```python
from build123d import *

# Parameters (mm, degrees)
SKETCH3_W           = 170.58
SKETCH3_H           = 100
BOSS_EXTRUDE1_DEPTH = 5
SKETCH4_W           = 5
SKETCH4_H           = 100
BOSS_EXTRUDE2_DEPTH = 24.94
SKETCH6_W           = 160.58
SKETCH6_H           = 5
BOSS_EXTRUDE3_DEPTH = 24.94
BOSS_EXTRUDE4_DEPTH = 24.94
SKETCH8_R           = 1.75
CUT_EXTRUDE1_DEPTH  = 8
SKETCH9_W           = 7.75
SKETCH9_H           = 6.74
CUT_EXTRUDE2_DEPTH  = 10
CUT_EXTRUDE3_DEPTH  = 10
SKETCH11_R          = 1.75
CUT_EXTRUDE4_DEPTH  = 10
SKETCH13_W          = 40.2
SKETCH13_H          = 14.565
CUT_EXTRUDE6_DEPTH  = 200
SKETCH14_R          = 1.75
CUT_EXTRUDE7_DEPTH  = 200
SKETCH15_R          = 1.5
CUT_EXTRUDE8_DEPTH  = 10
SKETCH16_R          = 1.75
CUT_EXTRUDE9_DEPTH  = 10


with BuildPart() as part:
    # Sketch3 → Boss-Extrude1 (new body)
    with BuildSketch(Plane(origin=(0, 0, 0), x_dir=(1, 0, 0), z_dir=(0, 1, 0))):
        with Locations((6.45008576, -36.464595487)):
            Rectangle(SKETCH3_W, SKETCH3_H)
    extrude(amount=BOSS_EXTRUDE1_DEPTH)

    # Sketch4 → Boss-Extrude2 (add)
    with BuildSketch(Plane(origin=(0, 5, 0), x_dir=(1, 0, 0), z_dir=(0, 1, 0))):
        with Locations((89.24008576, -36.464595487)):
            Rectangle(SKETCH4_W, SKETCH4_H)
        with Locations((-76.33991424, -36.464595487)):
            Rectangle(SKETCH4_W, SKETCH4_H)
    extrude(amount=BOSS_EXTRUDE2_DEPTH)

    # Sketch6 → Boss-Extrude3 (add)
    with BuildSketch(Plane(origin=(0, 5, 0), x_dir=(1, 0, 0), z_dir=(0, 1, 0))):
        with Locations((6.45008576, -83.964595487)):
            Rectangle(SKETCH6_W, SKETCH6_H)
    extrude(amount=BOSS_EXTRUDE3_DEPTH)

    # Sketch7 → Boss-Extrude4 (add)
    with BuildSketch(Plane(origin=(0, 5, 0), x_dir=(1, 0, 0), z_dir=(0, 1, 0))):
        Polygon((6.45008576, 13.535404513), (2.715085759, 13.535404513), (2.715085759, 8.535404513), (10.715085759, 8.535404513), (10.715085759, 13.535404513), align=None)
    extrude(amount=BOSS_EXTRUDE4_DEPTH)

    # Sketch8 → Cut-Extrude1 (cut)
    with BuildSketch(Plane.XY.offset(-8.535404513)):
        with Locations((6.715085759, 11.235)):
            Circle(SKETCH8_R)
        with Locations((6.715085759, 23.705)):
            Circle(SKETCH8_R)
    extrude(amount=-CUT_EXTRUDE1_DEPTH, mode=Mode.SUBTRACT)

    # Sketch9 → Cut-Extrude2 (cut)
    with BuildSketch(Plane.ZY.offset(78.83991424)):
        with Locations((-9.660404513, 26.57)):
            Rectangle(SKETCH9_W, SKETCH9_H)
    extrude(amount=-CUT_EXTRUDE2_DEPTH, mode=Mode.SUBTRACT)


with BuildPart() as body_2:
    # Mirror1: mirrored copy
    add(part.part.mirror(Plane(origin=(0, 29.94, 0), x_dir=(0, 0, 1), z_dir=(0, -1, 0))))

    # Sketch10 → Cut-Extrude3 (cut)
    with BuildSketch(Plane(origin=(0, 59.88, 0), x_dir=(1, 0, 0), z_dir=(0, 1, 0))):
        Polygon((16.71508576, -6.464595487), (6.45008576, -6.464595487), (-3.28491424, -6.464595487), (-3.28491424, -21.464595487), (16.71508576, -21.464595487), align=None)
    extrude(amount=-CUT_EXTRUDE3_DEPTH, mode=Mode.SUBTRACT)

    # Sketch11 → Cut-Extrude4 (cut)
    with BuildSketch(Plane(origin=(0, 59.88, 0), x_dir=(1, 0, 0), z_dir=(0, 1, 0))):
        with Locations(Location((-48.41990951, 0.535400876, 0), (0, 0, 270))):
            Circle(SKETCH11_R)
        with Locations(Location((-48.41990951, -7.464599124, 0), (0, 0, 270))):
            Circle(SKETCH11_R)
        with Locations(Location((61.31009049, -7.464599124, 0), (0, 0, 270))):
            Circle(SKETCH11_R)
        with Locations(Location((61.31009049, 0.535400876, 0), (0, 0, 270))):
            Circle(SKETCH11_R)
    extrude(amount=-CUT_EXTRUDE4_DEPTH, mode=Mode.SUBTRACT)

    # Sketch13 → Cut-Extrude6 (cut)
    with BuildSketch(Plane.ZY.offset(78.83991424)):
        with Locations((44.339595487, 37.2225)):
            Rectangle(SKETCH13_W, SKETCH13_H)
    extrude(amount=-CUT_EXTRUDE6_DEPTH, mode=Mode.SUBTRACT)

    # Sketch14 → Cut-Extrude7 (cut)
    with BuildSketch(Plane.ZY.offset(78.83991424)):
        with Locations((19.43959554, 35.1)):
            Circle(SKETCH14_R)
        with Locations((69.23959554, 35.1)):
            Circle(SKETCH14_R)
    extrude(amount=-CUT_EXTRUDE7_DEPTH, mode=Mode.SUBTRACT)

    # Sketch15 → Cut-Extrude8 (cut)
    with BuildSketch(Plane(origin=(0, 59.88, 0), x_dir=(1, 0, 0), z_dir=(0, 1, 0))):
        with Locations(Location((61.31009049, -83.964595487, 0), (0, 0, 270))):
            Circle(SKETCH15_R)
        with Locations(Location((-48.41990951, -83.964595487, 0), (0, 0, 270))):
            Circle(SKETCH15_R)
    extrude(amount=-CUT_EXTRUDE8_DEPTH, mode=Mode.SUBTRACT)

    # Sketch16 → Cut-Extrude9 (cut)
    with BuildSketch(Plane.XY.offset(86.464595487)):
        with Locations((21.687920531, 37.44)):
            Circle(SKETCH16_R)
        with Locations((-8.252079469, 37.44)):
            Circle(SKETCH16_R)
    extrude(amount=-CUT_EXTRUDE9_DEPTH, mode=Mode.SUBTRACT)


solid = body_2.part
```
Input: part model. Units: mm. Frame: model coordinates. A direction names the side the tool comes from. Coordinates: 2 decimals unless noted, no trailing zeros. Loops run counter-clockwise (first coordinate to the right, second up) from the corner with the lowest first, then second, coordinate; pieces in that order, holes last. Notation, with made-up numbers: M 3,-23 L 40,-23 A8 cw 40,-13 Z; hole C -24,17.25 d8. An arc over 180 degrees is marked long. Answer in a Markdown table with one row per item.
1. Draft query along X for faces 5 (the cylindrical face through (6.336, 50.353, -11)), 6 (the cylindrical face through (89.21, 33.55, 20.25)), 7 (the flat face through (91.74, 48, 37)). Return one class per face: pulls with the +X half, pulls with the -X half, needs draft (parallel to the pull), parting line crosses it, or undercut.
Response:
| item | result |
|---|---|
| face 5 | undercut |
| face 6 | needs draft |
| face 7 | pulls with the +X half |
2. Section A-A, the plane z = 30. Output: boundary loops of the cut face in (x, y) (3 decimals), then the cut area to 3 significant figures.
Response:
| item | result |
|---|---|
| outline | M -78.84,44.505 L -73.84,44.505 L -73.84,54.88 L 86.74,54.88 L 86.74,44.505 L 91.74,44.505 L 91.74,59.88 L -78.84,59.88 Z |
| area | 957 mm2 |
3. Material intervals for line 1 (X direction, y = 50, z = 73.5); line 2 (Z direction, x = 8.5, y = 40.75); line 3 (Y direction, x = 1.5, z = 51.5), sorted ascending.
Response:
| item | result |
|---|---|
| line 1 | x = -78.84 to -73.84, 86.74 to 91.74 |
| line 2 | z = -13.54 to -8.54, 81.46 to 86.46 |
| line 3 | y = 54.88 to 59.88 |
4. Section D-D, the plane z = 3. Output: boundary loops of the cut face in (x, y).
Response:
| item | result |
|---|---|
| outline | M -78.84,29.94 L -73.84,29.94 L -73.84,54.88 L 86.74,54.88 L 86.74,29.94 L 91.74,29.94 L 91.74,59.88 L -78.84,59.88 Z |
5. Reachability of faces 1 (the flat face through (-76, 44.505, 44)), 2 (the cylindrical face through (8.33, 36.85, -11)), 3 (the cylindrical face through (-47.969, 54.95, 85.395)), 4 (the flat face through (86.74, 45, 35)) from +Z, -Z, +X, -X, +Y, -Y: full face, straight path, thin tool, end or side. Return the list, or none.
Response:
| item | result |
|---|---|
| face 1 | +X, -X, -Y |
| face 2 | -Z |
| face 3 | +Y |
| face 4 | -Z, -Y |
6. Section C-C, the plane x = 44. Output: boundary loops of the cut face in (y, z), then the cut area to 3 significant figures.
Response:
| item | result |
|---|---|
| outline | M 29.94,81.46 L 54.88,81.46 L 54.88,-13.54 L 59.88,-13.54 L 59.88,86.46 L 29.94,86.46 Z |
| area | 625 mm2 |
7. First-contact query: pin 1 (4 mm diameter, centred on x = 58, y = 36, fed in from -Z); pin 2 (12 mm diameter, centred on x = 24, z = -2.5, fed in from -Y); pin 3 (5.5 mm diameter, centred on x = 90, z = 38.5, fed in from -Y) (3 decimals); pin 4 (5.5 mm diameter, centred on y = 35.1, z = 69.24, fed in from +X). Flat tips, straight axial feed; report the tip coordinate or a pass-through.
Response:
| item | result |
|---|---|
| pin 1 | stops at z = 81.46 |
| pin 2 | stops at y = 54.88 |
| pin 3 | stops at y = 44.505 |
| pin 4 | stops at x = 91.74 |
8. Section B-B, the plane y = 52.25. Output: boundary loops of the cut face in (x, z), then the cut area to 3 significant figures.
Response:
| item | result |
|---|---|
| outline | M -78.84,-13.54 L -73.84,-13.54 L -73.84,81.46 L 86.74,81.46 L 86.74,-13.54 L 91.74,-13.54 L 91.74,86.46 L -78.84,86.46 Z; M 2.72,-13.54 L 10.72,-13.54 L 10.72,-8.54 L 2.72,-8.54 Z; hole C -48.42,83.96 d3; hole C 61.31,83.96 d3 |
| area | 1,830 mm2 |
